The listing builds one solid part. Answer for the finished solid, in the listing's coordinates (mm). Face numbers are marked on the shaded views. A direction names the side the tool comes from. Coordinates: 2 decimals unless noted, no trailing zeros. Write each loop counter-clockwise with the first axis right and the second up, starting at its lowest first coordinate (ties: lowest second). Pieces come first, ordered by that corner, then holes.
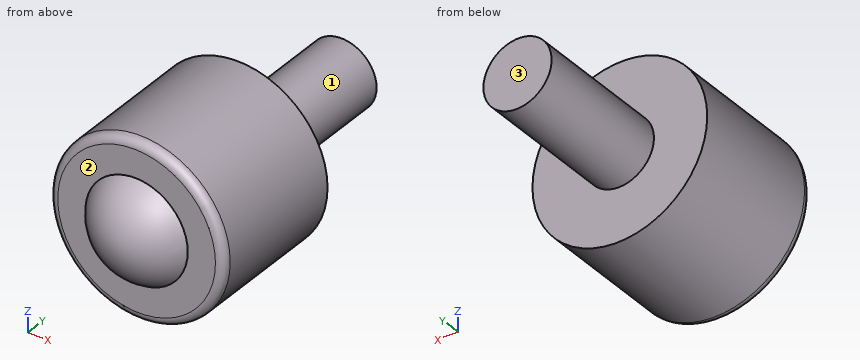
from build123d import *

# Parameters (mm, degrees)
CONG_1_R = 1


with BuildPart() as part:
    # Esquisse1 → Révolution1 (revolve)
    with BuildSketch(Plane.XY):
        with BuildLine():
            Line((10.25, 0), (6, 0))
            ThreePointArc((6, 0), (3.44818793, -2.490919876), (0, -3.4))
            Line((0, -3.4), (0, 0))
            Line((0, 0), (0, 33))
            Line((0, 33), (4, 33))
            Line((4, 33), (4, 16.6))
            Line((4, 16.6), (10.25, 16.6))
            Line((10.25, 16.6), (10.25, 0))
        make_face()
    revolve(axis=Axis((0, 33, 0), (0, -1, 0)))

    # Congé1
    cong_1_edges = [part.edges().sort_by_distance(p)[0] for p in [
        (-10.25, 0, 0),
    ]]
    fillet(cong_1_edges, radius=CONG_1_R)


solid = part.part
Q1. The part is cut by section C-C, the plane y = 28. Write down the section's boundary in (x, z), then the cut area to 3 significant figures.
Answers below:
outline: circle Ø8 at (0, 0)
area: 50.3 mm2
Q2. The part is cut by section B-B, the plane z = 0. Write down the section's boundary in (x, y), then the cut area to 3 significant figures.
Answers below:
outline: (-10.25, 1) arc R1 ccw to (-9.25, 0) - (-6, 0) arc R6.99 ccw to (6, 0) - (9.25, 0) arc R1 ccw to (10.25, 1) - (10.25, 16.6) - (4, 16.6) - (4, 33) - (-4, 33) - (-4, 16.6) - (-10.25, 16.6) - close
area: 500 mm2
Q3. The part is cut by section A-A, the plane x = 0. Write down the section's boundary in (y, z), then the cut area to 3 significant figures.
Answers below:
outline: (0, -9.25) arc R1 ccw to (1, -10.25) - (16.6, -10.25) - (16.6, -4) - (33, -4) - (33, 4) - (16.6, 4) - (16.6, 10.25) - (1, 10.25) arc R1 ccw to (0, 9.25) - (0, 6) arc R6.99 ccw to (0, -6) - close
area: 500 mm2
Q4. Which of the six approach directions +Z, -Z, +X, -X, +Y, -Y give full straight-line access (tool end or side, diameter ignored) to the marked faces 1, 2 and 3?
Answers below:
face 1: +Y
face 2: -Y
face 3: +Z, -Z, +X, -X, +Y
Q5. Find the intervals of material crossed by probe 1 along Y at (x, z) = (0, -8.5); probe 2 along X at (y, z) = (-2, -1); probe 3 along Z at (x, y) = (3.5, 22), in increasing order.
Answers below:
probe 1: y = 0 to 16.6
probe 2: x = -4.08 to 4.08
probe 3: z = -1.94 to 1.94
Q6. The part is cut by section D-D, the plane y = 5. Write down the section's boundary in (x, z).
Answers below:
outline: circle Ø20.5 at (0, 0)
Q7. Given pin 1 (1.5 mm diameter, centred on x = 4.5, z = 3.5, fed in from -Y); pin 2 (2 mm diameter, centred on x = 5, z = -3.5, fed in from -Y); pin 3 (1 mm diameter, centred on y = 11, z = 8, fed in from +X), each flat-ended and moving along its own axis, determine where each tip first touches the part or whether it passes through.
Answers below:
pin 1: stops at y = -1.35
pin 2: stops at y = -1.19
pin 3: stops at x = 6.99
